Geometry: final body of the model. Coordinates: model frame, mm. Give positions to 0.01 mm unless a question says otherwise; leave off trailing zeros. Loops run counter-clockwise (first coordinate to the right, second up) from the corner with the lowest first, then second, coordinate; pieces in that order, holes last. Notation, with made-up numbers: (-25.75, 28) - (2.25, 28) arc R15 cw to (2.25, 32) - close; hole circle Ø3 at (-4, 18.25). An arc over 180 degrees is marked (long way). Answer in a Markdown table with one row per item.
Autodesk Inventor part; units mm, degrees
ref_plane "YZ Plane" through (0, 0, 0) normal (1, 0, 0) x (0, 1, 0)
ref_plane "XZ Plane" through (0, 0, 0) normal (0, 1, 0) x (-1, 0, 0)
ref_plane "XY Plane" through (0, 0, 0) normal (0, 0, 1) x (1, 0, 0)
sketch "Schizzo2" plane through (0, 0, 0) normal (0, 0, 1) x (1, 0, 0)
  line L0 (-25, 47.5) -> (25, 47.5)
  line L1 (25, 47.5) -> (25, -47.5)
  line L2 (25, -47.5) -> (-25, -47.5)
  line L3 (-25, -47.5) -> (-25, 47.5)
  line L4 (-25, 47.5) -> (25, -47.5) construction
  line L5 (25, 47.5) -> (-25, -47.5) construction
  point P0 (0, 0)
  dimension "d0" = 50
  dimension "d1" = 95
extrude "Estrusione1" add sketch "Schizzo2" along normal blind 10
fillet "Raccordo1" radius 2 4 edges at (25, 47.5, 5) (-25, 47.5, 5) (25, -47.5, 5) (-25, -47.5, 5)
sketch "Schizzo3" plane through (0, 0, 0) normal (0, 0, -1) x (-1, 0, 0)
  line L0 (23, 47.5) -> (-23, 47.5)
  line L1 (25, -45.5) -> (25, 45.5)
  line L2 (-25, 45.5) -> (-25, -45.5)
  point P0 (0, 0)
  point P1 (15, 40.6)
  point P2 (-15, 40.6)
  dimension "d5" = 6.9
  dimension "d6" = 10
  dimension "d7" = 10
hole "Foro1" at (-15, 40.6, 0) at (15, 40.6, 0) direction (0, 0, 1) diameter 5.5 end through all countersink diameter 10.4 countersink angle 90
properties part number "Piastra sostegno asse"
Q1. First-contact query: pin 1 (5 mm diameter, centred on x = -15, y = 40.6, fed in from +Z). Flat tip, straight axial feed; report the tip coordinate or a pass-through.
Check values:
| item | result |
|---|---|
| pin 1 | through |
Q2. Cut plane A-A (x = -15). Output: boundary loops of the cut face in (y, z).
Check values:
| item | result |
|---|---|
| outline | (-47.5, 0) - (35.4, 0) - (37.85, 2.45) - (37.85, 10) - (-47.5, 10) - close; (43.35, 2.45) - (45.8, 0) - (47.5, 0) - (47.5, 10) - (43.35, 10) - close |
Q3. Draft query along Y for faces 1 (the cylindrical face through (14.879, 37.853, 6.278)), 2 (the flat face through (0, 1, 0)), 3 (the cylindrical face through (-24.43, -46.9, 5.07)). Return one class per face: pulls with the +Y half, pulls with the -Y half, needs draft (parallel to the pull), parting line crosses it, or undercut.
Check values:
| item | result |
|---|---|
| face 1 | undercut |
| face 2 | needs draft |
| face 3 | pulls with the -Y half |
Q4. Cut plane B-B (y = 40.6). Output: boundary loops of the cut face in (x, z).
Check values:
| item | result |
|---|---|
| outline | (-25, 0) - (-20.2, 0) - (-17.75, 2.45) - (-17.75, 10) - (-25, 10) - close; (-12.25, 2.45) - (-9.8, 0) - (9.8, 0) - (12.25, 2.45) - (12.25, 10) - (-12.25, 10) - close; (17.75, 2.45) - (20.2, 0) - (25, 0) - (25, 10) - (17.75, 10) - close |
Q5. Material intervals for line 1 along X through (y, z) = (40.6, 6.25); line 2 along Y through (x, z) = (15, 7); line 3 along X through (y, z) = (38.5, 0.75), sorted ascending.
Check values:
| item | result |
|---|---|
| line 1 | -25 to -17.75, -12.25 to 12.25, 17.75 to 25 |
| line 2 | -47.5 to 37.85, 43.35 to 47.5 |
| line 3 | -25 to -18.92, -11.08 to 11.08, 18.92 to 25 |
